Here's the drawing with two shaded views (mm, measured from the low corner). I have some questions. A direction names the side the tool comes from. Round coordinates to 2 decimals unless told otherwise and drop trailing zeros. Loops run counter-clockwise (first coordinate to the right, second up) from the corner with the lowest first, then second, coordinate; pieces in that order, holes last.
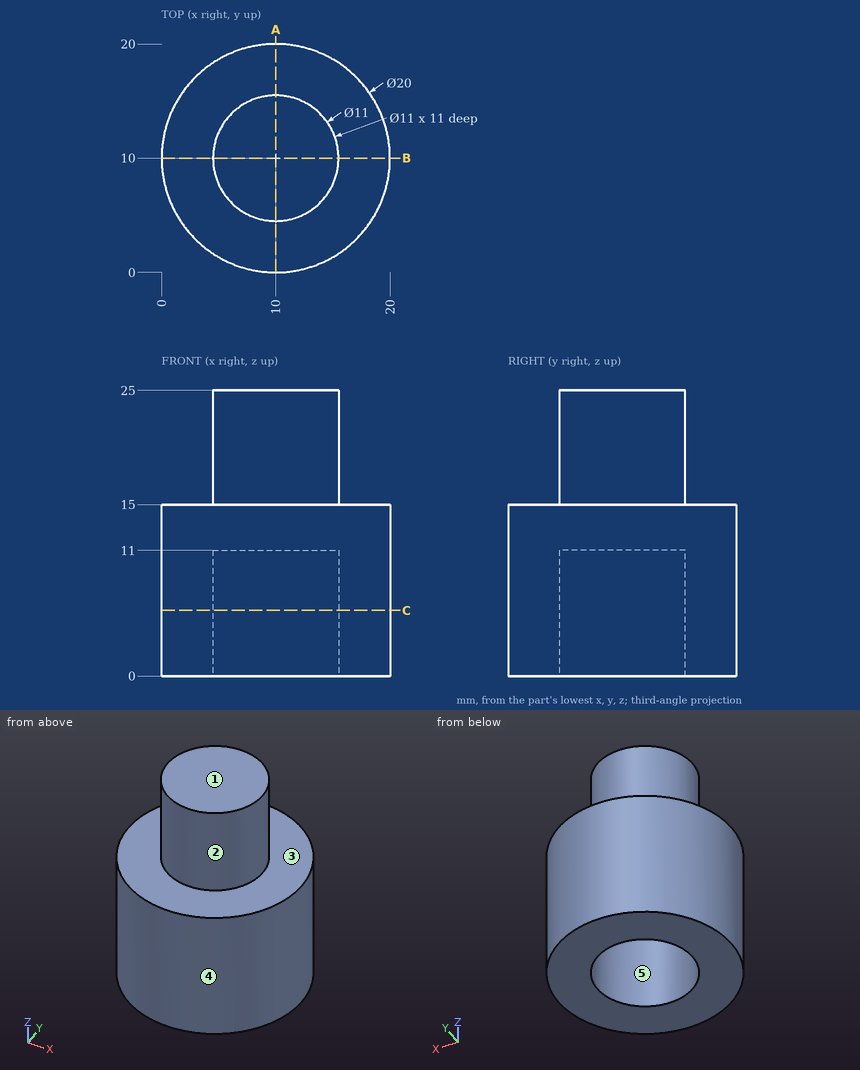
Item 1: If we section it at A-A, the plane x = 10: Please give me the cut outline in (y, z).
Results list:
outline: (0, 0) - (4.5, 0) - (4.5, 11) - (15.5, 11) - (15.5, 0) - (20, 0) - (20, 15) - (15.5, 15) - (15.5, 25) - (4.5, 25) - (4.5, 15) - (0, 15) - close
Item 2: We'd pull the mould along Y, two halves only. Please class the marked faces 3, 4 and 5: released by +Y, released by -Y, zero draft, split by the parting line, or undercut.
Results list:
face 3: zero draft
face 4: split by the parting line
face 5: undercut
Item 3: Will these pins go through, and if not, where does the flat tip stop? pin 1 (1 mm diameter, centred on y = 8, z = 8.5, fed in from +X); pin 2 (1.5 mm diameter, centred on x = 17, y = 17.5, fed in from -Z); pin 3 (5 mm diameter, centred on x = 15.5, z = 15.5, fed in from -Y); pin 4 (8 mm diameter, centred on x = 13.5, z = 22, fed in from +Y).
Results list:
pin 1: stops at x = 19.89
pin 2: stops at z = 0
pin 3: stops at y = 0.48
pin 4: stops at y = 15.5
Item 4: If I drill on line 1 along Y through (x, z) = (10, 5); line 2 along Z through (x, y) = (10.75, 9.5); line 3 along Z through (x, y) = (15.5, 5.75), over which ranges is the centre line in solid material (lowest first)?
Results list:
line 1: y = 0 to 4.5, 15.5 to 20
line 2: z = 11 to 25
line 3: z = 0 to 15
Item 5: If we section it at C-C, the plane z = 5.75: Please give me the cut outline in (x, y), then the cut area to 3 significant figures.
Results list:
outline: circle Ø20 at (10, 10); hole circle Ø11 at (10, 10)
area: 219 mm2
Item 6: For the marked faces 1 and 2, which set-ups out of +Z, -Z, +X, -X, +Y, -Y let a thin tool reach every point of the face, with its end or its side?
Results list:
face 1: +Z, +X, -X, +Y, -Y
face 2: +Z
